Autodesk Fusion 360 part; units mm, degrees
sketch "Sketch1" plane through (0, 0, 0) normal (0, 0, 1) x (1, 0, 0)
  line L0 (0, 0) -> (20, 0)
  line L1 (20, 0) -> (20, 45)
  line L2 (20, 45) -> (0, 45)
  line L3 (0, 45) -> (0, 0)
  circle A0 centre (9.8866, 34.5367) radius 8
  circle A1 centre (10.1679, 10.139) radius 8
  circle A2 centre (2, 43) radius 1
  circle A3 centre (18, 42) radius 1
  circle A4 centre (18, 2) radius 1
  circle A5 centre (2, 2) radius 1
  point P0 (2, 43)
  dimension "d1" = 20
  dimension "d2" = 45
  dimension "d3" = 16
  dimension "d4" = 16
extrude "Extrude1" add sketch "Sketch1" along normal blind 2
sketch "Sketch2" plane through (0, 0, 0) normal (1, 0, 0) x (0, 1, 0)
  line L0 (0, 0) -> (45, 0)
  line L1 (45, 0) -> (45, 15)
  line L2 (45, 15) -> (0, 15)
  line L3 (0, 15) -> (0, 0)
  circle A0 centre (3.2668, 7.4482) radius 2.5
  circle A1 centre (41.8901, 7.426) radius 2.5
  dimension "d7" = 5
  dimension "d8" = 5
extrude "Extrude2" add sketch "Sketch2" against normal blind 1
sketch "Sketch3" plane through (0, 0, 2) normal (0, 0, 1) x (-1, 0, 0)
  circle A0 centre (-2, -2) radius 1
  circle A1 centre (-18, -2) radius 1
  circle A2 centre (-10.1679, -10.139) radius 8
  circle A3 centre (-18, -42) radius 1
  circle A4 centre (-9.8866, -34.5367) radius 8
  circle A5 centre (-2, -43) radius 1
  line L0 (0, -45) -> (0, 0)
  line L1 (0, 0) -> (-20, 0)
  line L2 (-20, 0) -> (-20, -45)
  line L3 (-20, -45) -> (0, -45)
extrude "Extrude3" add 1 faces at (-1, 16.6085, 13.1343) along direction (-1, 0, 0) blind 3
extrude "Extrude4" add sketch "Sketch3" along normal blind 1
The listing builds one solid part. Answer for the finished solid, in the listing's coordinates (mm). A direction names the side the tool comes from. Coordinates: 2 decimals unless noted, no trailing zeros. Loops run counter-clockwise (first coordinate to the right, second up) from the corner with the lowest first, then second, coordinate; pieces in that order, holes last. Notation, with made-up numbers: (-40, 60.25) - (-23, 60.25) arc R32 cw to (-23, 89.25) - close; hole circle Ø3 at (-37, 58). An arc over 180 degrees is marked (long way). Use a Markdown table: item, result. Add a question column.
1) Find the intervals of material crossed by line 1 (X direction, y = 2, z = 1.2); line 2 (Y direction, x = -0.5, z = 7.25); line 3 (Y direction, x = 13, z = 2.5), in increasing order.
2) The part is cut by section C-C, the plane y = 19.5. Give the vertices of the cut face in (x, z), and give its area (3 significant figures).
3) The mould has two halves that part along Y. Classify faces 1 (the flat face through (2, 0, 2)), 2 (the flat face through (20, 22, 1)), 3 (the cylindrical face through (-1.97, 44.2, 6.47)), 4 (the flat face through (5, 45, 1)): released by +Y, released by -Y, zero draft, split by the parting line, or undercut.
4) The part is cut by section A-A, the plane x = 13.5. Give the vertices of the cut face in (y, z).
5) The part is cut by section B-B, the plane y = 29.5. Give the vertices of the cut face in (x, z), and give its area (3 significant figures).
6) Given pin 1 (3 mm diameter, centred on x = 8, y = 23, fed in from -Z); pin 2 (1.8 mm diameter, centred on x = 2, y = 43, fed in from -Z); pin 3 (4 mm diameter, centred on y = 35, z = 8.5, fed in from +X); pin 4 (3 mm diameter, centred on x = 13.5, y = 22.5, fed in from +Z), each flat-ended and moving along its own axis, determine where each tip first touches the part or whether it passes through.
7) The part is cut by section D-D, the plane x = 6.75. Give the vertices of the cut face in (y, z).
8) For faces 5 (the flat face through (0, 22, 9)), 6 (the cylindrical face through (-1.97, 4.42, 5.23)), determine the directions among +Z, -Z, +X, -X, +Y, -Y from which every point of the face is accessible in a straight line to the end or side of a thin tool.
Here are the results:
| question | item | result |
|---|---|---|
| 1 | line 1 | x = -4 to 1, 3 to 17, 19 to 20 |
| 1 | line 2 | y = 0 to 0.77, 5.76 to 39.4, 44.38 to 45 |
| 1 | line 3 | y = 0 to 2.66, 17.62 to 27.17, 41.91 to 45 |
| 2 | outline | (-4, 0) - (20, 0) - (20, 3) - (0, 3) - (0, 15) - (-4, 15) - close |
| 2 | area | 120 mm^2 |
| 3 | face 1 | released by -Y |
| 3 | face 2 | zero draft |
| 3 | face 3 | undercut |
| 3 | face 4 | released by +Y |
| 4 | outline | (0, 0) - (2.87, 0) - (2.87, 3) - (0, 3) - close; (17.41, 0) - (27.4, 0) - (27.4, 3) - (17.41, 3) - close; (41.67, 0) - (45, 0) - (45, 3) - (41.67, 3) - close |
| 5 | outline | (-4, 0) - (3.67, 0) - (3.67, 3) - (0, 3) - (0, 15) - (-4, 15) - close; (16.1, 0) - (20, 0) - (20, 3) - (16.1, 3) - close |
| 5 | area | 82.7 mm^2 |
| 6 | pin 1 | stops at z = 0 |
| 6 | pin 2 | passes through |
| 6 | pin 3 | stops at x = 0 |
| 6 | pin 4 | stops at z = 3 |
| 7 | outline | (0, 0) - (2.91, 0) - (2.91, 3) - (0, 3) - close; (17.37, 0) - (27.18, 0) - (27.18, 3) - (17.37, 3) - close; (41.9, 0) - (45, 0) - (45, 3) - (41.9, 3) - close |
| 8 | face 5 | +Z, +X, +Y, -Y |
| 8 | face 6 | +X, -X |
